Part model, mm, in its own coordinate system. Coordinates: 2 decimals unless noted, no trailing zeros. Write each loop counter-clockwise with the first axis right and the second up, starting at its lowest first coordinate (ties: lowest second). Pieces come first, ordered by that corner, then holes. Notation, with made-up numbers: (56.25, -27.75) -> (100.25, -27.75) arc R15 ccw to (100.25, -22.75) -> close; hole circle Ø3 at (81.25, 72.25). An arc over 180 degrees is marked (long way). Write item = value, one per line.
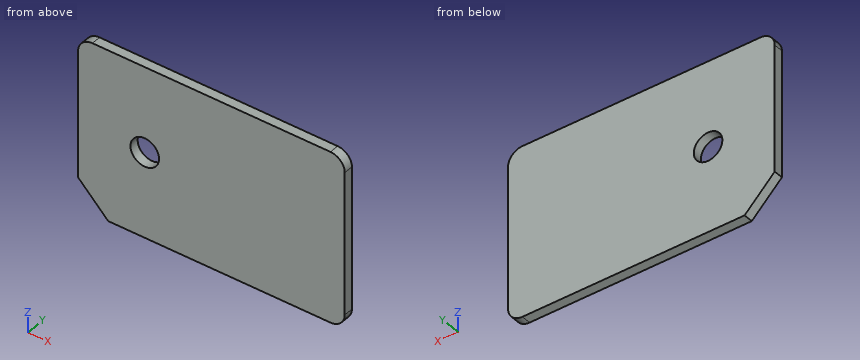
from build123d import *

# Parameters (mm, degrees)
BOSS_EXTRUDE1_DEPTH = 2
SKETCH3_R           = 2.999590147
CUT_EXTRUDE1_DEPTH  = 2


with BuildPart() as part:
    # Sketch1 → Boss-Extrude1 (new body)
    with BuildSketch(Plane(origin=(0, 0, 0), x_dir=(1, 0, 0), z_dir=(0, 1, 0))):
        with BuildLine():
            Line((-56.662746608, 29.55617923), (-50.334319483, 35.884606354))
            Line((-50.334319483, 35.884606354), (-3.662746608, 35.884606354))
            ThreePointArc((-3.662746608, 35.884606354), (-1.541426264, 35.005926698), (-0.662746608, 32.884606354))
            Line((-0.662746608, 32.884606354), (-0.662746608, 2.884606354))
            ThreePointArc((-0.662746608, 2.884606354), (-1.541426264, 0.763286011), (-3.662746608, -0.115393646))
            Line((-3.662746608, -0.115393646), (-53.662746608, -0.115393646))
            ThreePointArc((-53.662746608, -0.115393646), (-55.784066951, 0.763286011), (-56.662746608, 2.884606354))
            Line((-56.662746608, 2.884606354), (-56.662746608, 29.55617923))
        make_face()
    extrude(amount=BOSS_EXTRUDE1_DEPTH)

    # Sketch3 → Cut-Extrude1 (cut)
    with BuildSketch(Plane(origin=(0, 2, 0), x_dir=(1, 0, 0), z_dir=(0, 1, 0))):
        with Locations((-42.662746608, 17.884606354)):
            Circle(SKETCH3_R)
    extrude(amount=-CUT_EXTRUDE1_DEPTH, mode=Mode.SUBTRACT)


solid = part.part
Q1. Pin check, flat tip, straight feed: pin 1 (4 mm diameter, centred on x = -7, z = -6, fed in from -Y). Stop position of the tip, or through.
Model answer:
pin_1 = 0
Q2. Saw through at C-C on z = -32. Give the cut face in (x, y), and give its area (3 significant figures).
Model answer:
outline = (-54.22, 0) -> (-0.66, 0) -> (-0.66, 2) -> (-54.22, 2) -> close
area = 107 mm²
Q3. Saw through at B-B on x = -44.5. Give the cut face in (y, z).
Model answer:
outline = (0, -35.88) -> (2, -35.88) -> (2, -20.26) -> (0, -20.26) -> close; (0, -15.51) -> (2, -15.51) -> (2, 0.12) -> (0, 0.12) -> close
Q4. Saw through at A-A on y = 0.95. Give the cut face in (x, z).
Model answer:
outline = (-56.66, -29.56) -> (-50.33, -35.88) -> (-3.66, -35.88) arc R3 ccw to (-0.66, -32.88) -> (-0.66, -2.88) arc R3 ccw to (-3.66, 0.12) -> (-53.66, 0.12) arc R3 ccw to (-56.66, -2.88) -> close; hole circle Ø6 at (-42.66, -17.88)
Q5. Probe line 1 (X direction, y = 0.8, z = -16); line 2 (X direction, y = 0.65, z = -33). List the from-to ranges inside material, lowest first. Write a range as from..to.
Model answer:
line_1 = -56.66..-45, -40.33..-0.66
line_2 = -53.22..-0.66
